Source: CAD feature listing. Evaluate the final solid. Frame: model axes, mm. A direction names the side the tool comes from. Coordinates: 2 decimals unless noted, no trailing zeros. Loops run counter-clockwise (first coordinate to the right, second up) from the corner with the lowest first, then second, coordinate; pieces in that order, holes last.
Item 1: Line query: probe 1 along X at (y, z) = (0.25, 2.05); probe 2 along Z at (x, y) = (-8, 9.5); probe 3 along Y at (x, z) = (-2, 0.2). Output: solid intervals per line, ascending.
Item 2: Section query A-A, the plane y = 0. Return the cut outline in (x, z), then the cut area to 3 significant figures.
Item 3: Section query B-B, the plane x = -6.5. Return the cut outline in (y, z).
Item 4: Pin query (flat end, axial travel): pin 1 Ø1.5 at (x, z) = (-1.5, 3.5) entering from -Y; pin 2 Ø1 at (x, y) = (5.5, -4.5) entering from -Z; pin 3 Ø1 at (y, z) = (8.5, 1) entering from +X; pin 4 Ø1.5 at (y, z) = (-5, 2) entering from -X. Return the tip coordinate at first contact, or that it passes through.
Item 5: Section query C-C, the plane z = 3.75. Return the cut outline in (x, y).
Item 6: Reachability of faces 1 (the flat face through (8.5, 0, 3)), 2 (the flat face through (2, -2, 5)), 3 (the flat face through (0, 10, 2)) from +Z, -Z, +X, -X, +Y, -Y: full face, straight path, thin tool, end or side. Return the list, or none.
Item 7: Pull-direction query (X, two-part tool) for faces 4 (the cylindrical face through (4.38, -8.43, 3.48)), 5 (the flat face through (3, -3, 0)), 6 (the flat face through (-5, -0.75, 3)); classes: +X half, -X half, draft (parallel to the pull), parting line (faces both ways), or undercut.
```python
from build123d import *

# Parameters (mm, degrees)
OUTER_SKETCH_R           = 12.75
OUTER_DEPTH              = 2
INNER_SKETCH_R           = 9.5
INNER_DEPTH              = 3
CUT_OUT_SKETCH_W         = 7.75
CUT_OUT_SKETCH_H         = 1.5
CUT_OUT_SKETCH_W_2       = 1.5
CUT_OUT_SKETCH_H_2       = 7.75
ODEBRAT_VYSUNUT_M1_DEPTH = 19.711627401


with BuildPart() as part:
    # Outer sketch → Outer (new body)
    with BuildSketch(Plane.XY):
        Circle(OUTER_SKETCH_R)
    extrude(amount=OUTER_DEPTH)

    # Inner sketch → Inner (add)
    with BuildSketch(Plane.XY.offset(2)):
        Circle(INNER_SKETCH_R)
    extrude(amount=INNER_DEPTH)

    # Cut out sketch → Odebrat vysunutím1 (cut, through all)
    with BuildSketch(Plane.XY.offset(5)):
        with Locations((-4.625, 0)):
            Rectangle(CUT_OUT_SKETCH_W, CUT_OUT_SKETCH_H)
        with Locations((0, 4.625)):
            Rectangle(CUT_OUT_SKETCH_W_2, CUT_OUT_SKETCH_H_2)
        Rectangle(CUT_OUT_SKETCH_W_2, CUT_OUT_SKETCH_H)
        with Locations((0, -4.625)):
            Rectangle(CUT_OUT_SKETCH_W_2, CUT_OUT_SKETCH_H_2)
        with Locations((4.625, 0)):
            Rectangle(CUT_OUT_SKETCH_W, CUT_OUT_SKETCH_H)
    extrude(amount=-ODEBRAT_VYSUNUT_M1_DEPTH, mode=Mode.SUBTRACT)


solid = part.part
```
Verdict:
1. probe 1: x = -9.5 to -8.5, 8.5 to 9.5
1. probe 2: z = 0 to 2
1. probe 3: y = -12.59 to -0.75, 0.75 to 12.59
2. outline: (-12.75, 0) - (-8.5, 0) - (-8.5, 5) - (-9.5, 5) - (-9.5, 2) - (-12.75, 2) - close; (8.5, 0) - (12.75, 0) - (12.75, 2) - (9.5, 2) - (9.5, 5) - (8.5, 5) - close
2. area: 23.0 mm2
3. outline: (-10.97, 0) - (-0.75, 0) - (-0.75, 5) - (-6.93, 5) - (-6.93, 2) - (-10.97, 2) - close; (0.75, 0) - (10.97, 0) - (10.97, 2) - (6.93, 2) - (6.93, 5) - (0.75, 5) - close
4. pin 1: stops at y = -9.47
4. pin 2: stops at z = 0
4. pin 3: stops at x = 9.93
4. pin 4: stops at x = -12.02
5. outline: circle Ø19 at (0, 0); hole (-8.5, -0.75) - (-0.75, -0.75) - (-0.75, -8.5) - (0.75, -8.5) - (0.75, -0.75) - (8.5, -0.75) - (8.5, 0.75) - (0.75, 0.75) - (0.75, 8.5) - (-0.75, 8.5) - (-0.75, 0.75) - (-8.5, 0.75) - close
6. face 1: +Z, -Z
6. face 2: +Z, +X, -X, +Y, -Y
6. face 3: +Z
7. face 4: parting line
7. face 5: draft
7. face 6: undercut
